Could you check a few things on this model? Use its own coordinates, in mm. Face numbers are marked on the shaded views. A direction names the side the tool comes from. Coordinates: 2 decimals unless noted, no trailing zeros. Write each loop counter-clockwise with the first axis right and the second up, starting at its lowest first coordinate (ties: lowest second). Pieces come first, ordered by that corner, then holes.
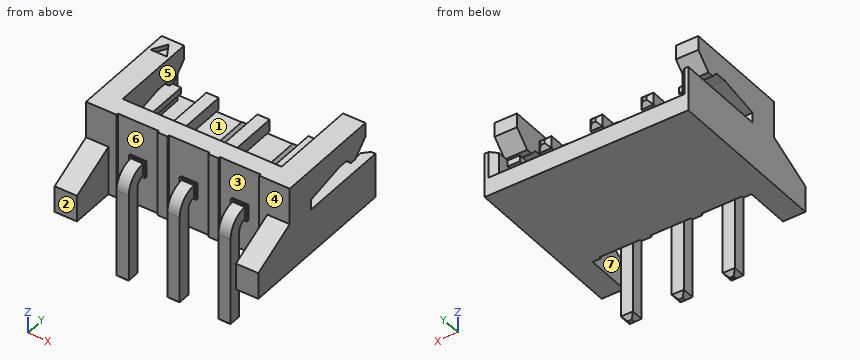
```python
from build123d import *

# Parameters (mm, degrees)
SKETCH_1_W                         = 10
SKETCH_1_H                         = 4.2
EXTRUDE_1_DEPTH                    = 6
CUT_EXTRUDE_1_DEPTH                = 5
CUT_EXTRUDE_2_DEPTH                = 13.395160346
EXTRUDE_6_DEPTH                    = 1.1
CUT_EXTRUDE_3_REACH                = 14.395
SKETCH_5_W                         = 7.8
SKETCH_5_H                         = 4.3
EXTRUDE_3_REACH                    = 13.995
EXTRUDE_5_REACH                    = 15.597
SKETCH_11_W                        = 2
SKETCH_11_H                        = 4.2
SKETCH_11_W_2                      = 0.8
SKETCH_11_H_2                      = 0.8
CUT_EXTRUDE_5_DEPTH                = 0.1
SKETCH_15_R                        = 0.05
CUT_EXTRUDE_6_DEPTH                = 0.1
PATTERN_LINEAR_2_COUNT             = 2
PATTERN_LINEAR_2_PITCH             = 2.5
CUT_EXTRUDE_7_DEPTH                = 0.2
SKETCH_7_W                         = 0.6
SKETCH_7_H                         = 0.6
EXTRUDE_4_DEPTH                    = 5.5
SKETCH_18_W                        = 0.6
SKETCH_18_H                        = 0.6
CHAMFER_6_SIZE                     = 0.2
PATTERN_LINEAR_1_COUNT             = 3
PATTERN_LINEAR_1_PITCH             = 2.5
CHAMFER_6_OF_PATTERN_LINEAR_1_SIZE = 0.2
CUT_EXTRUDE_4_REACH                = 13.995
SKETCH_20_W                        = 0.6
SKETCH_20_H                        = 0.3
CUT_EXTRUDE_9_DEPTH                = 0.9
CHAMFER_5_SIZE                     = 0.3
SKETCH_19_R                        = 0.05
CUT_EXTRUDE_8_DEPTH                = 3.2


with BuildPart() as part:
    # Эскиз1 → Бобышка-Вытянуть1 (new body)
    with BuildSketch(Plane(origin=(0, 0, 0), x_dir=(1, 0, 0), z_dir=(0, 1, 0))):
        with Locations((5, -2.1)):
            Rectangle(SKETCH_1_W, SKETCH_1_H)
    extrude(amount=EXTRUDE_1_DEPTH)

    # Эскиз2 → Вырез-Вытянуть1 (cut)
    with BuildSketch(Plane(origin=(0, 6, 0), x_dir=(1, 0, 0), z_dir=(0, 1, 0))):
        Polygon((0.5, -0.9), (9.5, -0.9), (9.5, -1.9), (8.9, -1.9), (8.9, -3.7), (1.1, -3.7), (1.1, -1.9), (0.5, -1.9), align=None)
    extrude(amount=-CUT_EXTRUDE_1_DEPTH, mode=Mode.SUBTRACT)

    # Эскиз3 → Вырез-Вытянуть2 (cut, through all)
    with BuildSketch(Plane.ZY):
        Polygon((2.2, 6), (2.2, 1.5), (2.7, 1.5), (3.1, 3.459591794), (3.1, 4.021282026), (2.8, 4.285857157), (2.8, 4.585857157), (3.5, 5.3), (4.2, 5.3), (4.2, 6), align=None)
    extrude(amount=-CUT_EXTRUDE_2_DEPTH, mode=Mode.SUBTRACT)

    # Эскиз16 → Бобышка-Вытянуть6 (add)
    with BuildSketch(Plane(origin=(10, 0, 0), x_dir=(0, 0, -1), z_dir=(1, 0, 0))):
        Polygon((-2.4, 0), (-1.3, -2.2), (0, -2.2), (0, 0), align=None)
    extrude_6 = extrude(amount=-EXTRUDE_6_DEPTH)

    # Зеркальное отражение2: Бобышка-Вытянуть6 across plane
    add(extrude_6.mirror(Plane(origin=(5, 0, 0), x_dir=(0, 0, 1), z_dir=(1, 0, 0))))

    # Эскиз5 → Вырез-Вытянуть3 (cut, up to next)
    with BuildSketch(Plane.XY.offset(4.2), mode=Mode.PRIVATE) as cut_extrude_3_sk1:
        with Locations((5, 3.15)):
            Rectangle(SKETCH_5_W, SKETCH_5_H)
    cut_extrude_3_tool1 = extrude(cut_extrude_3_sk1.sketch, amount=-CUT_EXTRUDE_3_REACH, mode=Mode.PRIVATE) & part.part
    add(cut_extrude_3_tool1.solids().sort_by_distance((5, 3.15, 4.2))[0], mode=Mode.SUBTRACT)

    # Эскиз6 → Бобышка-Вытянуть3 (add, up to next)
    with BuildSketch(Plane(origin=(0.5, 0, 0), x_dir=(0, 0, -1), z_dir=(1, 0, 0)), mode=Mode.PRIVATE) as extrude_3_sk1:
        Polygon((-3.3, 1), (-2.67, 1.5), (-0.9, 1.5), (-0.9, 1), align=None)
    extrude_3_tool1 = extrude(extrude_3_sk1.sketch, amount=EXTRUDE_3_REACH, mode=Mode.PRIVATE) - part.part
    add(extrude_3_tool1.solids().sort_by_distance((0.5, 1.23741, 1.950432))[0])

    # Эскиз9 → Бобышка-Вытянуть5 (add, up to next)
    with BuildSketch(Plane(origin=(0, 6, 0), x_dir=(1, 0, 0), z_dir=(0, 1, 0)), mode=Mode.PRIVATE) as extrude_5_sk1:
        Polygon((3.45, -0.9), (3.75, -1.328444402), (4.05, -0.9), align=None)
    extrude_5_tool1 = extrude(extrude_5_sk1.sketch, amount=-EXTRUDE_5_REACH, mode=Mode.PRIVATE) - part.part
    extrude_5 = extrude_5_tool1.solids().sort_by_distance((3.75, 6, 1.042815))[0]
    add(extrude_5)

    # Эскиз11 → Вырез-Вытянуть5 (cut)
    with BuildSketch(Plane.XZ):
        with Locations((2.5, 2.1)):
            Rectangle(SKETCH_11_W, SKETCH_11_H)
        with Locations((2.5, 2)):
            Rectangle(SKETCH_11_W_2, SKETCH_11_H_2, mode=Mode.SUBTRACT)
    cut_extrude_5 = extrude(amount=-CUT_EXTRUDE_5_DEPTH, mode=Mode.SUBTRACT)

    # Эскиз15 → Вырез-Вытянуть6 (cut)
    with BuildSketch(Plane.XZ):
        with Locations(Location((2.5, 2, 0), (0, 0, 270))):
            Circle(SKETCH_15_R)
    extrude(amount=-CUT_EXTRUDE_6_DEPTH, mode=Mode.SUBTRACT)

    # Линейный массив2: Бобышка-Вытянуть5 ×2
    with Locations(*[(i * PATTERN_LINEAR_2_PITCH, 0, 0) for i in range(1, PATTERN_LINEAR_2_COUNT)]):
        add(extrude_5)

    # Эскиз17 → Вырез-Вытянуть7 (cut)
    with BuildSketch(Plane.XY.offset(4.2)):
        Polygon((0.55, 5), (0.15, 4.307179677), (0.95, 4.307179677), align=None)
    extrude(amount=-CUT_EXTRUDE_7_DEPTH, mode=Mode.SUBTRACT)

    # Эскиз7 → Бобышка-Вытянуть4 (add)
    with BuildSketch(Plane.XZ):
        with Locations((2.5, 2)):
            Rectangle(SKETCH_7_W, SKETCH_7_H)
    extrude_4 = extrude(amount=-EXTRUDE_4_DEPTH)

    # По траектории1: sweep along a curve in space
    with BuildLine() as sweep_1_path:
        Line((2.5, -0.7, 1.3), (2.5, -0.7, -3.2))
        ThreePointArc((2.5, 0, 2), (2.5, -0.494974747, 1.794974747), (2.5, -0.7, 1.3))
    # Эскиз18 → По траектории1 (sweep)
    with BuildSketch(Plane.XZ):
        with Locations((2.5, 2)):
            Rectangle(SKETCH_18_W, SKETCH_18_H)
    sweep_1 = sweep(path=sweep_1_path.line)

    # Фаска6
    chamfer_6_edges = [part.edges().sort_by_distance(p)[0] for p in [
        (2.8, 5.5, 2),
        (2.5, 5.5, 1.7),
        (2.2, 5.5, 2),
        (2.5, 5.5, 2.3),
        (2.8, -0.7, -3.2),
        (2.5, -1, -3.2),
        (2.2, -0.7, -3.2),
        (2.5, -0.4, -3.2),
    ]]
    chamfer(chamfer_6_edges, length=CHAMFER_6_SIZE)

    # Линейный массив1: Вырез-Вытянуть5, Бобышка-Вытянуть4, По траектории1 ×3
    with Locations(*[(i * PATTERN_LINEAR_1_PITCH, 0, 0) for i in range(1, PATTERN_LINEAR_1_COUNT)]):
        add(cut_extrude_5, mode=Mode.SUBTRACT)
        add(extrude_4)
        add(sweep_1)

    # Фаска6 of Линейный массив1
    chamfer_6_of_pattern_linear_1_edges = [part.edges().sort_by_distance(p)[0] for p in [
        (5.3, 5.5, 2),
        (5, 5.5, 1.7),
        (4.7, 5.5, 2),
        (5, 5.5, 2.3),
        (5.3, -0.7, -3.2),
        (5, -1, -3.2),
        (4.7, -0.7, -3.2),
        (5, -0.4, -3.2),
        (7.8, 5.5, 2),
        (7.5, 5.5, 1.7),
        (7.2, 5.5, 2),
        (7.5, 5.5, 2.3),
        (7.8, -0.7, -3.2),
        (7.5, -1, -3.2),
        (7.2, -0.7, -3.2),
        (7.5, -0.4, -3.2),
    ]]
    chamfer(chamfer_6_of_pattern_linear_1_edges, length=CHAMFER_6_OF_PATTERN_LINEAR_1_SIZE)

    # Вырез-Вытянуть4: up to this face of the body (flat: up to its plane)
    cut_extrude_4_end = Plane(part.part.faces().sort_by_distance((9.5, 3.75, 1.4))[0])
    # Эскиз10 → Вырез-Вытянуть4 (cut, up to the picked face)
    with BuildSketch(Plane(origin=(0.5, 0, 0), x_dir=(0, 0, -1), z_dir=(1, 0, 0)), mode=Mode.PRIVATE) as cut_extrude_4_sk1:
        Polygon((-1.4, 6), (-0.9, 6), (-1.4, 5.5), align=None)
    cut_extrude_4_tool1 = split(extrude(cut_extrude_4_sk1.sketch, amount=CUT_EXTRUDE_4_REACH, mode=Mode.PRIVATE), bisect_by=cut_extrude_4_end, keep=Keep.BOTH, mode=Mode.PRIVATE)
    add(cut_extrude_4_tool1.solids().sort_by(Axis((0.5, 5.833333, 1.233333), (1, 0, 0)))[0], mode=Mode.SUBTRACT)

    # Эскиз20 → Вырез-Вытянуть9 (cut)
    with BuildSketch(Plane(origin=(0, 6, 0), x_dir=(1, 0, 0), z_dir=(0, 1, 0))):
        with Locations((0.8, -2.05)):
            Rectangle(SKETCH_20_W, SKETCH_20_H)
    cut_extrude_9 = extrude(amount=-CUT_EXTRUDE_9_DEPTH, mode=Mode.SUBTRACT)

    # Зеркальное отражение3: Вырез-Вытянуть9 across plane
    add(cut_extrude_9.mirror(Plane(origin=(5, 0, 0), x_dir=(0, 0, 1), z_dir=(1, 0, 0))), mode=Mode.SUBTRACT)

    # Фаска5
    chamfer_5_edges = [part.edges().sort_by_distance(p)[0] for p in [
        (0.5, 6, 1.55),
        (9.5, 6, 1.55),
    ]]
    chamfer(chamfer_5_edges, length=CHAMFER_5_SIZE)

    # Эскиз19 → Вырез-Вытянуть8 (cut)
    with BuildSketch(Plane(origin=(0, 0, 0), x_dir=(-1, 0, 0), z_dir=(0, 0, -1))):
        with Locations(Location((-2.5, -0.7, 0), (0, 0, 270))):
            Circle(SKETCH_19_R)
    extrude(amount=CUT_EXTRUDE_8_DEPTH, mode=Mode.SUBTRACT)


solid = part.part
```
1. I want a section at A-A on z = -2.25. Please give me the cut outline in (x, y), plus the area to 3 significant figures.
Verdict:
outline: (2.2, -1) - (2.8, -1) - (2.8, -0.4) - (2.2, -0.4) - close; (4.7, -1) - (5.3, -1) - (5.3, -0.4) - (4.7, -0.4) - close; (7.2, -1) - (7.8, -1) - (7.8, -0.4) - (7.2, -0.4) - close; hole circle Ø0.1 at (2.5, -0.7)
area: 1.07 mm2
2. On a 3-axis mill with a long thin cutter (end or side, diameter ignored), from which of +Z, -Z, +X, -X, +Y, -Y can I reach the whole of each face in a straight line? I mean the marked faces 4, 5, 6 and 7. Say none if no direction works.
Verdict:
face 4: +Z, -Y
face 5: +Z, +Y
face 6: none
face 7: +Z, -Z, -Y
3. If we mould it in two halves opening along Y, with no side actions, what happens to the marked faces 1, 2 and 3? For each: pulls with the +Y half, pulls with the -Y half, needs draft (parallel to the pull), parting line crosses it, or undercut.
Verdict:
face 1: needs draft
face 2: pulls with the -Y half
face 3: undercut
4. I want a section at B-B on z = 0.25. Give the number of separate pieces and of enclosed holes in the cut face, plus the area to 3 significant figures.
Verdict:
separate pieces: 4
enclosed holes: 0
area: 65.3 mm2
5. Please list where these lines run through material, in increasing order: line 1 along X through (y, z) = (-0.5, 1); line 2 along Z through (x, y) = (2.5, 4.5); line 3 along X through (y, z) = (1.5, 3.5).
Verdict:
line 1: x = 0 to 1.1, 2.2 to 2.8, 4.7 to 5.3, 7.2 to 7.8, 8.9 to 10
line 2: z = 0 to 0.9, 1.7 to 2.3
line 3: x = 0 to 1.1, 8.9 to 10
6. I want a section at C-C on x = 8.25. Please give me the cut outline in (y, z), plus the area to 3 significant figures.
Verdict:
outline: (0.1, 0) - (6, 0) - (6, 0.9) - (1.5, 0.9) - (1.5, 2.67) - (1, 3.3) - (1, 4.2) - (0.1, 4.2) - close
area: 9.32 mm2
7. For pin 1 (3 mm diameter, centred on x = 6, y = 4, fed in from -Z); pin 2 (0.8 mm diameter, centred on y = -0.5, z = -1, fed in from +X), each with a flat end and sliding along its axis, tell me the tip position at first contact or that it passes through.
Verdict:
pin 1: stops at z = 0
pin 2: stops at x = 7.8
8. I want a section at D-D on y = 0.75. Please give me the cut outline in (x, z), plus the area to 3 significant figures.
Verdict:
outline: (0, 0) - (10, 0) - (10, 4.2) - (0, 4.2) - close
area: 42.0 mm2
